from build123d import *

# Parameters (mm, degrees)
SKETCH1_R           = 22.225
BOSS_EXTRUDE1_DEPTH = 7.62
SKETCH2_R           = 2.413
CUT_EXTRUDE1_DEPTH  = 33.341392209
EXTRUDE_THIN1_DEPTH = 7.62
FILLET1_R           = 1.27


with BuildPart() as part:
    # Sketch1 → Boss-Extrude1 (new body)
    with BuildSketch(Plane.XY):
        with Locations(Location((0, 0, 0), (0, 0, 180))):
            Circle(SKETCH1_R)
    extrude(amount=BOSS_EXTRUDE1_DEPTH)

    # Sketch2 → Cut-Extrude1 (cut, through all)
    with BuildSketch(Plane.XY.offset(7.62)):
        Circle(SKETCH2_R)
        with BuildLine():
            Line((11.546285712, 9.679232711), (10.236925711, 6.871301126))
            ThreePointArc((10.236925711, 6.871301126), (10.277852612, 5.933920972), (11.069184188, 5.429787159))
            Line((11.069184188, 5.429787159), (14.155604273, 5.159760391))
            ThreePointArc((14.155604273, 5.159760391), (15.068334078, 5.577769607), (15.176404699, 6.575831801))
            ThreePointArc((15.176404699, 6.575831801), (14.323882769, 8.269897573), (13.28303974, 9.855236107))
            ThreePointArc((13.28303974, 9.855236107), (12.364657215, 10.260675301), (11.546285712, 9.679232711))
        make_face()
        with BuildLine():
            Line((2.609318561, -14.838993102), (0.832258477, -12.301088285))
            ThreePointArc((0.832258477, -12.301088285), (0, -11.867841944), (-0.832258477, -12.301088285))
            Line((-0.832258477, -12.301088285), (-2.609318561, -14.838993102))
            ThreePointArc((-2.609318561, -14.838993102), (-2.703676863, -15.838444908), (-1.893364959, -16.431067908))
            ThreePointArc((-1.893364959, -16.431067908), (0, -16.539795145), (1.893364959, -16.431067908))
            ThreePointArc((1.893364959, -16.431067908), (2.703676863, -15.838444908), (2.609318561, -14.838993102))
        make_face()
        with BuildLine():
            Line((-14.155604273, 5.159760391), (-11.069184188, 5.429787159))
            ThreePointArc((-11.069184188, 5.429787159), (-10.277852612, 5.933920972), (-10.236925711, 6.871301126))
            Line((-10.236925711, 6.871301126), (-11.546285712, 9.679232711))
            ThreePointArc((-11.546285712, 9.679232711), (-12.364657215, 10.260675301), (-13.28303974, 9.855236107))
            ThreePointArc((-13.28303974, 9.855236107), (-14.323882769, 8.269897573), (-15.176404699, 6.575831801))
            ThreePointArc((-15.176404699, 6.575831801), (-15.068334078, 5.577769607), (-14.155604273, 5.159760391))
        make_face()
        with BuildLine():
            ThreePointArc((7.245790098, 15.538647009), (0, 17.145), (-7.245790098, 15.538647009))
            ThreePointArc((-7.245790098, 15.538647009), (-9.580075747, 9.125249897), (-3.166678635, 6.790964248))
            ThreePointArc((-3.166678635, 6.790964248), (0, 7.493), (3.166678635, 6.790964248))
            ThreePointArc((3.166678635, 6.790964248), (9.580075747, 9.125249897), (7.245790098, 15.538647009))
        make_face()
        with BuildLine():
            ThreePointArc((9.833968001, -14.044361799), (14.848005548, -8.5725), (17.079758099, -1.494285209))
            ThreePointArc((17.079758099, -1.494285209), (12.6927361, 3.733964018), (7.464486873, -0.65305798))
            ThreePointArc((7.464486873, -0.65305798), (6.489128351, -3.7465), (4.297808238, -6.137906268))
            ThreePointArc((4.297808238, -6.137906268), (3.112660354, -12.859213915), (9.833968001, -14.044361799))
        make_face()
        with BuildLine():
            ThreePointArc((-17.079758099, -1.494285209), (-14.848005548, -8.5725), (-9.833968001, -14.044361799))
            ThreePointArc((-9.833968001, -14.044361799), (-3.112660354, -12.859213915), (-4.297808238, -6.137906268))
            ThreePointArc((-4.297808238, -6.137906268), (-6.489128351, -3.7465), (-7.464486873, -0.65305798))
            ThreePointArc((-7.464486873, -0.65305798), (-12.6927361, 3.733964018), (-17.079758099, -1.494285209))
        make_face()
    extrude(amount=-CUT_EXTRUDE1_DEPTH, mode=Mode.SUBTRACT)

    # Sketch3 → Extrude-Thin1 (add)
    with BuildSketch(Plane.XY.offset(7.62)):
        Polygon((0.635, 6.223), (0.635, 7.493), (0.635, 17.145), (-0.635, 17.145), (-0.635, 7.493), (-0.635, 6.223), align=None)
        Polygon((5.071776088, -3.661426131), (6.171628351, -4.296426131), (14.530505548, -9.122426131), (15.165505548, -8.022573869), (6.806628351, -3.196573869), (5.706776088, -2.561573869), align=None)
        Polygon((-5.706776088, -2.561573869), (-6.806628351, -3.196573869), (-15.165505548, -8.022573869), (-14.530505548, -9.122426131), (-6.171628351, -4.296426131), (-5.071776088, -3.661426131), align=None)
    extrude(amount=-EXTRUDE_THIN1_DEPTH)

    # Fillet1
    fillet1_edges = [part.edges().sort_by_distance(p)[0] for p in [
        (-0.635, 17.133236705, 3.81),
        (0.635, 17.133236705, 3.81),
        (0.635, 7.466044736, 3.81),
        (-0.635, 7.466044736, 3.81),
        (15.155318236, -8.016692221, 3.81),
        (14.520318236, -9.116544484, 3.81),
        (6.148284407, -4.282948499, 3.81),
        (6.783284407, -3.183096237, 3.81),
        (-14.520318236, -9.116544484, 3.81),
        (-15.155318236, -8.016692221, 3.81),
        (-6.783284407, -3.183096237, 3.81),
        (-6.148284407, -4.282948499, 3.81),
    ]]
    fillet(fillet1_edges, radius=FILLET1_R)


solid = part.part
Design review of the part built by this model. Coordinates are the model's own, in mm. A direction names the side the tool comes from. Give positions to 0.01 mm unless a question says otherwise; leave off trailing zeros. Loops run counter-clockwise (first coordinate to the right, second up) from the corner with the lowest first, then second, coordinate; pieces in that order, holes last. Notation, with made-up numbers: (5.25, 65) -> (60.25, 65) arc R14 ccw to (60.25, 82) -> close; hole circle Ø6 at (-7.5, 53.25). An arc over 180 degrees is marked (long way). One line per question, with ' | ' between items. Start each with the question number.
(1) We need section C-C (y = 13.5). State the section outline as (x, z) points (3 decimals).
(2) We need section D-D (z = 3.5). State how many separate pieces and enclosed holes the cut face has, and give its area (3 significant figures).
(3) We need section B-B (y = 0). State the section outline as (x, z) points (3 decimals), and give its area (3 significant figures).
(4) Insertion check: P1, Ø3.5, axis at y = 10.5, z = 5.5, coming from the +X side; P2, Ø3, axis at x = 0, y = 0, coming from the -Z side; P3, Ø3, axis at y = 8.5, z = 4.5, coming from the -X side; P4, Ø3.5, axis at y = 14, z = 5.5, coming from the -X side. Each pin has a flat end and moves straight along its axis. Give the tip position at first contact, or say it passes through.
(5) Draft analysis for pull direction X (two halves, no side actions). For faces 1 (the face through (-14.31, 8.29, 3.86)), 2 (the face through (0, 5, 7.62)), state which applies: +X half, -X half, draft (parallel to the pull), parting line (faces both ways), or undercut.
(6) For faces 3 (the face through (-0.03, -16.54, 3.86)), 4 (the face through (0, 5, 0)), list the 3-axis set-ups (+Z, -Z, +X, -X, +Y, -Y) from which the entire face can be reached by the end or side of a thin tool; tool diameter is ignored.
(7) For line 1 (X direction, y = -4.5, z = 3.5); line 2 (Y direction, x = -5, z = 5.5); line 3 (X direction, y = 13.5, z = 6) (3 decimals), list the stretches that pass through material, from the lowest coordinate up.
(8) We need section A-A (x = 0). State the section outline as (y, z) points (3 decimals), and give its area (3 significant figures).
The answers:
1) outline: (-17.655, 0) -> (-9.43, 0) -> (-9.43, 7.62) -> (-17.655, 7.62) -> close; (-0.635, 0) -> (0.635, 0) -> (0.635, 7.62) -> (-0.635, 7.62) -> close; (9.43, 0) -> (17.655, 0) -> (17.655, 7.62) -> (9.43, 7.62) -> close
2) separate pieces: 1 | enclosed holes: 10 | area: 990 mm^2
3) outline: (-22.225, 0) -> (-16.977, 0) -> (-16.977, 7.62) -> (-22.225, 7.62) -> close; (-7.567, 0) -> (-2.413, 0) -> (-2.413, 7.62) -> (-7.567, 7.62) -> close; (2.413, 0) -> (7.567, 0) -> (7.567, 7.62) -> (2.413, 7.62) -> close; (16.977, 0) -> (22.225, 0) -> (22.225, 7.62) -> (16.977, 7.62) -> close | area: 159 mm^2
4) P1: stops at x = 20.43 | P2: passes through | P3: stops at x = -21.09 | P4: stops at x = -18.54
5) face 1: undercut | face 2: draft
6) face 3: +Z, -Z | face 4: -Z, +X, -X, +Y, -Y
7) line 1: x = -21.76 to -16.54, -9.06 to 9.06, 16.54 to 21.76 | line 2: y = -21.66 to -14.45, -5.58 to 6.34, 16.4 to 21.66 | line 3: x = -17.655 to -9.43, -0.635 to 0.635, 9.43 to 17.655
8) outline: (-22.225, 0) -> (-16.54, 0) -> (-16.54, 7.62) -> (-22.225, 7.62) -> close; (-11.868, 0) -> (-2.413, 0) -> (-2.413, 7.62) -> (-11.868, 7.62) -> close; (2.413, 0) -> (22.225, 0) -> (22.225, 7.62) -> (2.413, 7.62) -> close | area: 266 mm^2
